For this review, use the dimensioned drawing (mm, ordinates from the lowest corner) and the shaded views. Round coordinates to 2 decimals unless told otherwise and drop trailing zeros. Write each loop counter-clockwise with the first axis right and the second up, starting at its lowest first coordinate (ties: lowest second). Pieces come first, ordered by that corner, then holes.
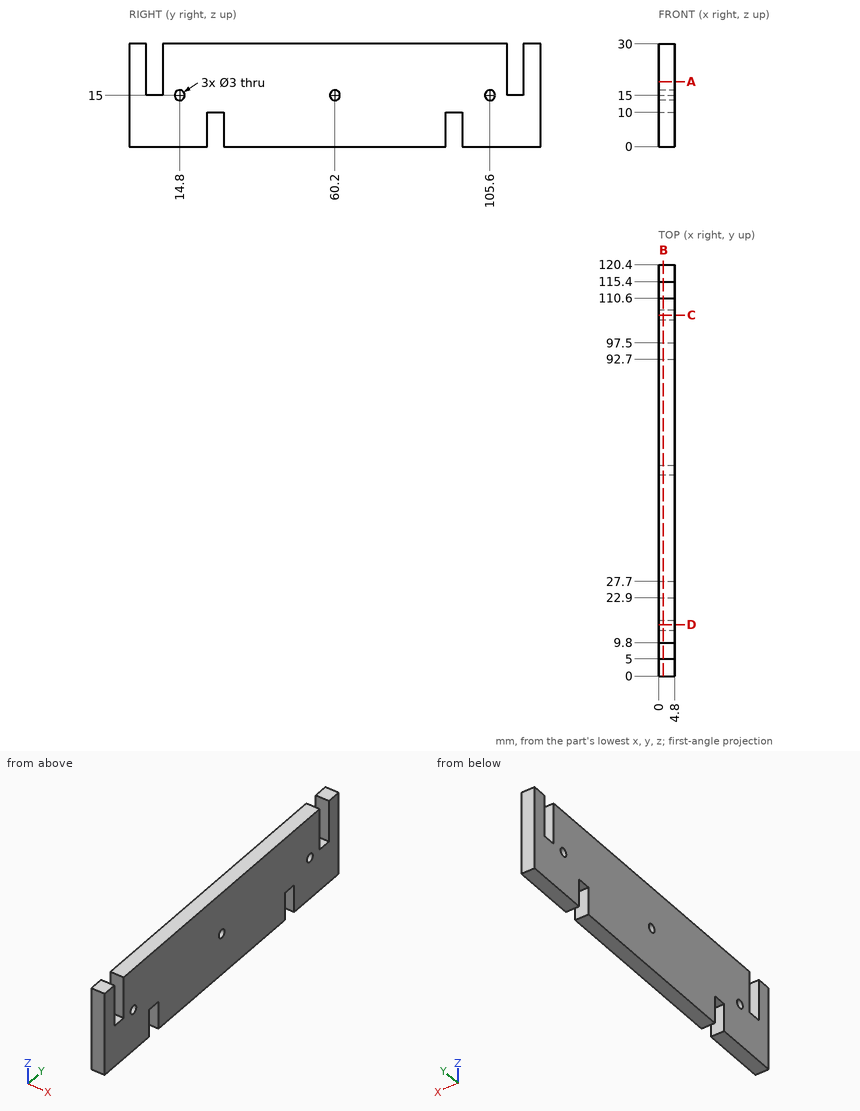
1) Add section D-D on y = 15. State the section outline as (x, z) points.
2) Add section C-C on y = 105.6. State the section outline as (x, z) points, and give its area (3 significant figures).
3) For line 1 along Y through (x, z) = (2.8, 20.75); line 2 along Y through (x, z) = (2.8, 8); line 3 along Z through (x, y) = (3.45, 105.6), list the stretches that pass through material, from the lowest coordinate up.
4) For P1, Ø2.5, axis at x = 2, y = 114, coming from the +Z side; P2, Ø1.5, axis at x = 0.5, y = 24.5, coming from the -Z side, all flat-tipped, find the tip position at first contact; note any pin that passes through.
5) Add section B-B on x = 1.4. State the section outline as (y, z) points.
6) Add section A-A on z = 19. State the section outline as (x, y) points.
Computed:
1. outline: (0, 0) - (4.8, 0) - (4.8, 13.51) - (0, 13.51) - close; (0, 16.49) - (4.8, 16.49) - (4.8, 30) - (0, 30) - close
2. outline: (0, 0) - (4.8, 0) - (4.8, 13.5) - (0, 13.5) - close; (0, 16.5) - (4.8, 16.5) - (4.8, 30) - (0, 30) - close
2. area: 130 mm2
3. line 1: y = 0 to 5, 9.8 to 110.6, 115.4 to 120.4
3. line 2: y = 0 to 22.9, 27.7 to 92.7, 97.5 to 120.4
3. line 3: z = 0 to 13.5, 16.5 to 30
4. P1: stops at z = 15
4. P2: stops at z = 10
5. outline: (0, 0) - (22.9, 0) - (22.9, 10) - (27.7, 10) - (27.7, 0) - (92.7, 0) - (92.7, 10) - (97.5, 10) - (97.5, 0) - (120.4, 0) - (120.4, 30) - (115.4, 30) - (115.4, 15) - (110.6, 15) - (110.6, 30) - (9.8, 30) - (9.8, 15) - (5, 15) - (5, 30) - (0, 30) - close; hole circle Ø3 at (14.8, 15); hole circle Ø3 at (60.2, 15); hole circle Ø3 at (105.6, 15)
6. outline: (0, 0) - (4.8, 0) - (4.8, 5) - (0, 5) - close; (0, 9.8) - (4.8, 9.8) - (4.8, 110.6) - (0, 110.6) - close; (0, 115.4) - (4.8, 115.4) - (4.8, 120.4) - (0, 120.4) - close
